Source: CAD feature listing. Evaluate the final solid. Frame: model axes, mm. Give positions to 0.01 mm unless a question says otherwise; leave off trailing zeros. Use CSV: the item, a comma, the result in double quotes.
```python
from build123d import *

# Parameters (mm, degrees)
SKETCH1_W                  = 650
SKETCH1_H                  = 253.35
BOSS_EXTRUDE1_DEPTH        = 20
FILLET1_R                  = 10
F_4_0_4_DIAMETER_HOLE1_D   = 4
F_7_0_7_DIAMETER_HOLE1_D   = 7
F_11_0_11_DIAMETER_HOLE1_D = 11
M8_CLEARANCE_HOLE1_D       = 8.4
M8_CLEARANCE_HOLE1_DEPTH   = 30
M8_CLEARANCE_HOLE1_TIP     = 2.5236146


with BuildPart() as part:
    # Sketch1 → Boss-Extrude1 (new body)
    with BuildSketch(Plane(origin=(0, 0, 0), x_dir=(1, 0, 0), z_dir=(0, 1, 0))):
        with Locations((325, 126.675)):
            Rectangle(SKETCH1_W, SKETCH1_H)
    extrude(amount=BOSS_EXTRUDE1_DEPTH)

    # Fillet1
    fillet1_edges = [part.edges().sort_by_distance(p)[0] for p in [
        (0, 10, 0),
        (0, 10, -253.35),
        (650, 10, -253.35),
        (650, 10, 0),
    ]]
    fillet(fillet1_edges, radius=FILLET1_R)

    # Ø4.0 (4) Diameter Hole1 (through all)
    with Locations(Plane(origin=(0, 20, 0), x_dir=(1, 0, 0), z_dir=(0, 1, 0))):
        with Locations((90.058331561, 195.482500532), (255.538984983, 64.732354618), (396.503986047, 162.794964053), (544.959880887, 152.580108904), (534.745025737, 49.750567065), (278.011666312, 162.794964053), (102.997148083, 96.05791041), (429.191522525, 213.869239801), (424.424590122, 108.315736589), (197.654805802, 187.310616412)):
            Hole(F_4_0_4_DIAMETER_HOLE1_D / 2)

    # Ø7.0 (7) Diameter Hole1 (through all)
    with Locations(Plane(origin=(0, 20, 0), x_dir=(1, 0, 0), z_dir=(0, 1, 0))):
        with Locations((128.874781129, 145.089215127), (77.119515038, 44.302644319), (325.680990343, 106.953755902), (340.662777896, 209.102307398), (502.057489259, 121.935543455), (570.156523589, 196.163490875), (588.543262858, 55.879480155)):
            Hole(F_7_0_7_DIAMETER_HOLE1_D / 2)

    # Ø11.0 (11) Diameter Hole1 (through all)
    with Locations(Plane(origin=(0, 20, 0), x_dir=(1, 0, 0), z_dir=(0, 1, 0))):
        with Locations((209.912631982, 116.487620709), (425.786570809, 41.578682945), (489.799663079, 194.120519845), (309.337222104, 41.578682945), (163.605288637, 46.345615349), (159.519346577, 220.679143234), (275.968695282, 220.679143234), (589.224253201, 120.573562769)):
            Hole(F_11_0_11_DIAMETER_HOLE1_D / 2)

    # M8 Clearance Hole1
    with Locations(Plane(origin=(0, 20, 0), x_dir=(1, 0, 0), z_dir=(0, 1, 0))):
        with Locations((25, 126.675), (625, 126.675)):
            Hole(M8_CLEARANCE_HOLE1_D / 2, depth=M8_CLEARANCE_HOLE1_DEPTH)
            with Locations((0, 0, -(M8_CLEARANCE_HOLE1_DEPTH + M8_CLEARANCE_HOLE1_TIP / 2))):  # 118° drill point
                Cone(0, M8_CLEARANCE_HOLE1_D / 2, M8_CLEARANCE_HOLE1_TIP, mode=Mode.SUBTRACT)


solid = part.part
```
1. Ray query, line 1 along Z through (x, y) = (589.5, 18.5); line 2 along X through (y, z) = (7.75, -162); line 3 along X through (y, z) = (6, -43). Return the intervals inside material, ascending.
Answer below:
line 1,"z = -253.35 to -126.07, -115.08 to -59.25, -52.51 to 0"
line 2,"x = 0 to 276.18, 279.85 to 394.67, 398.34 to 650"
line 3,"x = 0 to 73.87, 80.37 to 159.24, 167.97 to 304.02, 314.65 to 420.47, 431.1 to 650"
2. Mould query, pull axis X, two halves, no side actions, for faces 1 (the flat face through (0, 10, -125)), 2 (the cylindrical face through (154.273, 9.86, -222.331)), 3 (the flat face through (320, 0, -128)), 4 (the flat face through (650, 10, -125)). Classes: released by +X, released by -X, zero draft, split by the parting line, or undercut.
Answer below:
face 1,"released by -X"
face 2,"undercut"
face 3,"zero draft"
face 4,"released by +X"
3. Pin query (flat end, axial travel): P1, Ø7.5, axis at x = 25, z = -126.675, coming from the +Y side. Return the tip coordinate at first contact, or that it passes through.
Answer below:
P1,"passes through"
